from build123d import *

# Parameters (mm, degrees)
F1_DEPTH = 31.75
F3_DEPTH = 25.4
F5_DEPTH = 12.7
F7_DEPTH = 12.7


with BuildPart() as f1:
    # F0 (on Top) → F1 (new body)
    with BuildSketch(Plane.XY):
        Polygon((0, 31.75), (0, 0), (12.7, 0), (12.7, -25.4), (25.4, -25.4), (25.4, 0), (38.1, 0), (38.1, 31.75), align=None)
    extrude(amount=F1_DEPTH)

    # F2 (on face) → F3 (cut)
    with BuildSketch(Plane(origin=(12.7, 0, 0), x_dir=(0, -1, 0), z_dir=(-1, 0, 0))):
        Polygon((25.4, 31.75), (12.7, 31.75), (25.4, 0), align=None)
    extrude(amount=-F3_DEPTH, mode=Mode.SUBTRACT)

    # F4 (on face) → F5 (cut)
    with BuildSketch(Plane(origin=(0, 0, 0), x_dir=(0, -1, 0), z_dir=(-1, 0, 0))):
        Polygon((0, 31.75), (-15.875, 31.75), (0, 0), align=None)
    extrude(amount=-F5_DEPTH, mode=Mode.SUBTRACT)

    # F6 (on face) → F7 (cut)
    with BuildSketch(Plane.YZ.offset(38.1)):
        Polygon((0, 0), (15.875, 31.75), (0, 31.75), align=None)
    extrude(amount=-F7_DEPTH, mode=Mode.SUBTRACT)


solid = f1.part
Input: part model. Units: mm. Frame: model coordinates. A direction names the side the tool comes from. Round coordinates to 2 decimals unless told otherwise and drop trailing zeros. Write each loop counter-clockwise with the first axis right and the second up, starting at its lowest first coordinate (ties: lowest second). Pieces come first, ordered by that corner, then holes.
1) Draft query along Z for faces 1 (the flat face through (19, 10, 0)), 2 (the flat face through (32, 8, 16)), 3 (the flat face through (12.7, -4, 16)). Return one class per face: pulls with the +Z half, pulls with the -Z half, needs draft (parallel to the pull), parting line crosses it, or undercut.
2) Cut plane B-B (z = 19). Return the cut outline in (x, y), then the cut area to 3 significant figures.
3) Cut plane C-C (x = 3.5). Return the cut outline in (y, z) (3 decimals), then the cut area to 3 significant figures.
4) Cut plane D-D (y = -16.5). Return the cut outline in (x, z).
5) Contact query for a flat-ended pin moving along its axis: P1, Ø6, axis at y = -9.5, z = 4, coming from the +X side. Output: stop coordinate, or through.
6) Ray query, L1, parallel to X at y = 2, z = 21.5; L2, parallel to Z at x = 26, y = 8.5; L3, parallel to Y at x = 8, z = 16. Return the intervals inside material, ascending.
7) Cut plane A-A (y = 15). Return the cut outline in (x, z), then the cut area to 3 significant figures.
8) Reachability of faces 4 (the flat face through (25.4, -5, 16)), 5 (the flat face through (19, 31.75, 16)), 6 (the flat face through (6, 8, 16)) from +Z, -Z, +X, -X, +Y, -Y: full face, straight path, thin tool, end or side. Return the list, or none.
Geometry says:
1. face 1: pulls with the -Z half
1. face 2: pulls with the +Z half
1. face 3: needs draft
2. outline: (0, 9.5) - (12.7, 9.5) - (12.7, -17.8) - (25.4, -17.8) - (25.4, 9.5) - (38.1, 9.5) - (38.1, 31.75) - (0, 31.75) - close
2. area: 1,190 mm2
3. outline: (0, 0) - (31.75, 0) - (31.75, 31.75) - (15.875, 31.75) - close
3. area: 756 mm2
4. outline: (12.7, 0) - (25.4, 0) - (25.4, 22.25) - (12.7, 22.25) - close
5. P1: stops at x = 25.4
6. L1: x = 12.7 to 25.4
6. L2: z = 0 to 17
6. L3: y = 8 to 31.75
7. outline: (0, 0) - (38.1, 0) - (38.1, 30) - (25.4, 30) - (25.4, 31.75) - (12.7, 31.75) - (12.7, 30) - (0, 30) - close
7. area: 1,170 mm2
8. face 4: +Z, +X, -Y
8. face 5: +Z, -Z, +X, -X, +Y
8. face 6: +Z, -X, -Y
